from build123d import *

# Parameters (mm, degrees)
SKETCH1_R                = 14.312899999999999
BOSS_EXTRUDE1_DEPTH      = 6.35
FILLET1_R                = 14.2875
SKETCH2_W                = 63.5
SKETCH2_H                = 38.099999999999994
BOSS_EXTRUDE2_DEPTH      = 6.35
FILLET2_R                = 14.2875
SKETCH5_W                = 80.56082205671558
SKETCH5_H                = 59.96207335790194
CUT_EXTRUDE3_DEPTH       = 105.34114720473416
SKETCH6_R                = 14.312899999999999
BOSS_EXTRUDE3_DEPTH      = 88.89999999999999
CHAMFER1_SIZE            = 123.334861862
CHAMFER1_SIZE_2          = 86.36
CHAMFER2_START           = -41.62371919
CHAMFER2_OUTLINE_W       = 158.00000000000003
CHAMFER2_OUTLINE_H       = 88.9
CHAMFER2_DEPTH           = 70.741970545
BOSS_EXTRUDE4_DEPTH      = 6.35
BOSS_EXTRUDE5_DEPTH      = 73.65999999999998
CUT_EXTRUDE9_DEPTH       = 140.7047508401556
CUT_EXTRUDE9_DEPTH_BACK  = 140.7047508401556
CUT_EXTRUDE10_DEPTH      = 73.65999999999998
CUT_EXTRUDE10_DEPTH_BACK = 184.87947802715968
FILLET3_R                = 20.16
SKETCH19_R               = 2.539999999999996
CUT_EXTRUDE11_DEPTH      = 184.87947795602068
SKETCH20_R               = 2.5400000000000027
SKETCH20_R_2             = 2.540000000000001
CUT_EXTRUDE12_DEPTH      = 188.65942191717963
FILLET4_R                = 20.16
CUT_EXTRUDE13_DEPTH      = 330.8952367610784
CUT_EXTRUDE13_DEPTH_BACK = 330.8952367610784
SKETCH21_W               = 304.0212933781311
SKETCH21_H               = 127.80861110845143


with BuildPart() as part:
    # Sketch1 → Boss-Extrude1 (new body)
    with BuildSketch(Plane.XY):
        Polygon((-6.34999999999998, -6.349999999999993), (63.500000000000014, -6.349999999999988), (63.50000000000003, 44.44999999999999), (-63.49999999999997, 44.44999999999999), (-63.49999999999994, -44.45), (-31.749999999999943, -44.45), align=None)
        with Locations((-44.44999999999997, -25.400000000000006)):
            Circle(SKETCH1_R, mode=Mode.SUBTRACT)
        with Locations((35.87185256827684, 12.70000000000001)):
            Circle(SKETCH1_R, mode=Mode.SUBTRACT)
    extrude(amount=BOSS_EXTRUDE1_DEPTH)

    # Fillet1
    fillet1_edges = [part.edges().sort_by_distance(p)[0] for p in [
        (-31.749999999999943, -44.45, 3.175),
        (-63.49999999999994, -44.45, 3.175),
        (63.50000000000002, -6.349999999999987, 3.175),
        (-6.349999999999981, -6.349999999999993, 3.175),
    ]]
    fillet(fillet1_edges, radius=FILLET1_R)

    # Sketch2 → Boss-Extrude2 (add)
    with BuildSketch(Plane.XY.offset(6.35)):
        with Locations((2.842e-14, 63.499999999999986)):
            Rectangle(SKETCH2_W, SKETCH2_H)
    extrude(amount=-BOSS_EXTRUDE2_DEPTH)

    # Fillet2
    fillet2_edges = [part.edges().sort_by_distance(p)[0] for p in [
        (-31.74999999999997, 82.54999999999998, 3.175),
        (31.75000000000003, 82.54999999999998, 3.175),
        (31.75000000000003, 44.44999999999999, 3.175),
    ]]
    fillet(fillet2_edges, radius=FILLET2_R)

    # Sketch5 → Cut-Extrude3 (cut, through all)
    with BuildSketch(Plane.XY.offset(6.35)):
        with Locations((8.530411028357818, 74.43103667895096)):
            Rectangle(SKETCH5_W, SKETCH5_H)
    extrude(amount=-CUT_EXTRUDE3_DEPTH, mode=Mode.SUBTRACT)

    # Sketch6 → Boss-Extrude3 (add)
    # profile 1 of 2: a face of its own
    with BuildSketch(Plane.XY.offset(6.35)):
        with BuildLine():
            Line((-27.50851936904525, -38.08777905356794), (49.21250000000003, -6.349999999999989))
            Line((49.21250000000003, -6.349999999999989), (1.296437949397273, -6.3499999999999925))
            ThreePointArc((1.296437949397273, -6.3499999999999925), (-5.445232161641531, -8.040574170103001), (-10.591480630954672, -12.71222094643204))
            Line((-10.591480630954672, -12.71222094643204), (-27.50851936904525, -38.08777905356794))
        make_face()
    # profile 2 of 2: a face of its own
    with BuildSketch(Plane.XY.offset(6.35)):
        with BuildLine():
            ThreePointArc((49.21250000000003, -6.349999999999989), (59.315288136202824, -2.1652881362027863), (63.50000000000003, 7.937500000000011))
            Line((63.50000000000003, 7.937500000000011), (63.50000000000003, 44.44999999999999))
            Line((63.50000000000003, 44.44999999999999), (-63.49999999999997, 44.44999999999999))
            Line((-63.49999999999997, 44.44999999999999), (-63.49999999999994, -30.162500000000005))
            ThreePointArc((-63.49999999999994, -30.162500000000005), (-59.31528813620274, -40.2652881362028), (-49.21249999999995, -44.45))
            Line((-49.21249999999995, -44.45), (-39.396437949397196, -44.45))
            ThreePointArc((-39.396437949397196, -44.45), (-32.65476783835839, -42.759425829897), (-27.50851936904525, -38.08777905356794))
            Line((-27.50851936904525, -38.08777905356794), (-10.591480630954672, -12.71222094643204))
            ThreePointArc((-10.591480630954672, -12.71222094643204), (-5.445232161641531, -8.040574170103001), (1.296437949397273, -6.3499999999999925))
            Line((1.296437949397273, -6.3499999999999925), (49.21250000000003, -6.349999999999989))
        make_face()
        with Locations((35.87185256827684, 12.70000000000001)):
            Circle(SKETCH6_R, mode=Mode.SUBTRACT)
        with Locations((-44.44999999999997, -25.400000000000006)):
            Circle(SKETCH6_R, mode=Mode.SUBTRACT)
    extrude(amount=-BOSS_EXTRUDE3_DEPTH)

    # Chamfer1
    # the kernel refuses this chamfer: 123.334861862, 86.36 mm, written as the material it takes off along each edge
    with BuildSketch(Plane(origin=(63.50000000000003, -310.58122257411287, -82.55), x_dir=(-1, 0, 0), z_dir=(0, 1, 0))) as chamfer1_piece_1:
        Polygon((CHAMFER1_SIZE, 0), (0, CHAMFER1_SIZE_2), (0, 0), align=None)
    extrude(amount=673.5499451482258, mode=Mode.SUBTRACT)

    # Chamfer2: read off the stored shape, not the designer's step
    # Chamfer2 outline → Chamfer2 (cut)
    with BuildSketch(Plane(origin=(0, 0, 0), x_dir=(0.819152044288991, 0, 0.5735764363510472), z_dir=(0.5735764363510472, 0, -0.8191520442889911)).offset(CHAMFER2_START)):
        with Locations((-22.000000000000004, 0)):
            Rectangle(CHAMFER2_OUTLINE_W, CHAMFER2_OUTLINE_H)
    extrude(amount=CHAMFER2_DEPTH, mode=Mode.SUBTRACT)

    # Sketch8 → Boss-Extrude4 (add)
    with BuildSketch(Plane(origin=(63.50000000000003, 0, 0), x_dir=(0, 0, -1), z_dir=(1, 0, 0))):
        Polygon((-3.8100000000002296, 44.44999999999999), (-41.91000000000023, 44.44999999999998), (-41.910000000000224, 7.937500000000005), (-3.8100000000002257, 7.937500000000011), align=None)
    extrude(amount=-BOSS_EXTRUDE4_DEPTH)

    # Sketch10 → Boss-Extrude5 (add)
    with BuildSketch(Plane(origin=(0, 44.44999999999999, 0), x_dir=(1, 0, 0), z_dir=(0, 1, 0))):
        Polygon((-57.84497848897024, 130.81000000000014), (-63.49999999999997, 130.81000000000014), (-63.49999999999997, 80.01000000000018), (-57.844978488970234, 80.01000000000016), align=None)
    extrude(amount=-BOSS_EXTRUDE5_DEPTH)

    # Sketch17 → Cut-Extrude9 (cut, two sides: drawn at the far end of the back side and taken through both)
    with BuildSketch(Plane(origin=(19.10074600681286, 0, -27.278692336917096), x_dir=(-0.8191520442889909, 0, -0.5735764363510474), z_dir=(0.5735764363510474, 0, -0.8191520442889909)).offset(-CUT_EXTRUDE9_DEPTH_BACK)):
        with BuildLine():
            add(Edge.make_bspline(
                [(94.42353448054058, -29.21), (95.93788750756819, -24.718047698019056), (93.93338517829203, -20.356820676396385)],
                knots=[2.872150837356143, 2.872150837356143, 2.872150837356143, 3.5016757767347815, 3.5016757767347815, 3.5016757767347815], degree=2, weights=[1, 0.9508699428937519, 1]))
            add(Edge.make_bspline(
                [(93.93338517829203, -20.356820676396385), (88.79622683458668, -9.179825042266891), (74.45226902252679, -11.318450120374129), (60.108311210466894, -13.457075198481366), (60.108311210466894, -25.4)],
                knots=[3.5016757767347815, 3.5016757767347815, 3.5016757767347815, 4.892430541957184, 4.892430541957184, 6.283185307179586, 6.283185307179586, 6.283185307179586], degree=2, weights=[1, 0.7678119767762641, 1, 0.7678119767762641, 1]))
            add(Edge.make_bspline(
                [(60.108311210466894, -25.400000000000002), (60.108311210466894, -37.903779229296156), (75.2342951684929, -39.58320874739981), (90.36027912651893, -41.262638265503455), (94.42353448054058, -29.21)],
                knots=[0, 0, 0, 1.4360754186780715, 1.4360754186780715, 2.872150837356143, 2.872150837356143, 2.872150837356143], degree=2, weights=[1, 0.7530981852489751, 1, 0.7530981852489751, 1]))
        make_face()
    extrude(amount=CUT_EXTRUDE9_DEPTH + CUT_EXTRUDE9_DEPTH_BACK, mode=Mode.SUBTRACT)

    # Sketch18 → Cut-Extrude10 (cut, two sides: drawn at the far end of the back side and taken through both)
    with BuildSketch(Plane(origin=(-57.84497848897023, 0, 7.9e-15), x_dir=(-1.4e-16, 0, -1), z_dir=(1, 0, -1.4e-16)).offset(-CUT_EXTRUDE10_DEPTH_BACK)):
        Polygon((130.81000000000014, -29.21), (81.15666866187213, -29.210000000000008), (81.15666866187213, -3.8100000000000076), (130.81000000000014, -3.810000000000001), align=None)
    extrude(amount=CUT_EXTRUDE10_DEPTH + CUT_EXTRUDE10_DEPTH_BACK, mode=Mode.SUBTRACT)

    # Fillet3
    # the kernel refuses this fillet: 20.16 mm, written as the material it adds along each edge
    with BuildSketch(Plane(origin=(57.150000000000034, 44.44999999999999, 4.470039485332174), x_dir=(-0.8191520442889912, 0, -0.5735764363510469), z_dir=(0, -1, 0))) as fillet3_piece_1_section:
        with BuildLine():
            CenterArc((FILLET3_R * 0.520567050552, -FILLET3_R), FILLET3_R, 90.00000000000001, 54.99999999999993)
            Line((-FILLET3_R * 0.298584993737, -FILLET3_R * 0.426423563649), (0, 0))
            Line((0, 0), (FILLET3_R * 0.520567050552, 0))
        make_face()
    fillet3_piece_1 = extrude(amount=36.51249999999998, mode=Mode.PRIVATE)
    fillet3_piece_1 = fillet3_piece_1 - Plane(origin=(35.87185256827684, 12.70000000000001, 4.470039485332174), x_dir=(1, 0, 0), z_dir=(0, 0, 1)) * Cylinder(14.312899999999999, 116, mode=Mode.PRIVATE)
    add(fillet3_piece_1)
    with BuildSketch(Plane(origin=(-57.844978488970234, 44.44999999999999, -81.15666866204359), x_dir=(0.8191520442884476, 0, 0.5735764363518233), z_dir=(0, -1, 0))) as fillet3_piece_2:
        with BuildLine():
            CenterArc((FILLET3_R * 0.520567050551, -FILLET3_R), FILLET3_R, 90.00000000000001, 54.99999999994567)
            Line((-FILLET3_R * 0.298584993737, -FILLET3_R * 0.426423563648), (0, 0))
            Line((0, 0), (FILLET3_R * 0.520567050551, 0))
        make_face()
    extrude(amount=48.25999999999999)

    # Sketch19 → Cut-Extrude11 (cut, through all)
    with BuildSketch(Plane(origin=(-57.84497848897023, 0, 7.9e-15), x_dir=(-1.4e-16, 0, -1), z_dir=(1, 0, -1.4e-16))):
        with Locations((121.28500000000014, 28.57499999999999)):
            Circle(SKETCH19_R)
        with Locations((121.28500000000014, 5.7149999999999945)):
            Circle(SKETCH19_R)
    extrude(amount=-CUT_EXTRUDE11_DEPTH, mode=Mode.SUBTRACT)

    # Sketch20 → Cut-Extrude12 (cut, through all)
    with BuildSketch(Plane(origin=(63.50000000000003, 0, 0), x_dir=(0, 0, -1), z_dir=(1, 0, 0))):
        with Locations((-32.38500000000023, 25.39999999999998)):
            Circle(SKETCH20_R)
        with Locations((-16.510000000000232, 25.399999999999977)):
            Circle(SKETCH20_R_2)
    extrude(amount=-CUT_EXTRUDE12_DEPTH, mode=Mode.SUBTRACT)

    # Fillet4
    # the kernel refuses this fillet: 20.16 mm, written as the material it takes off along each edge
    with BuildSketch(Plane(origin=(-41.42329156376277, -29.209999999999994, -82.55), x_dir=(0, -2.04e-14, 1), z_dir=(-1, 0, 0))) as fillet4_piece_1:
        with BuildLine():
            CenterArc((20.160000000000146, -7.364628119294481), FILLET4_R, 158.57340370727903, 21.426596292722138)
            Line((1.5023e-13, -7.364628119294892), (-0.403199999999848, -7.3646281192949))
            Line((-0.403199999999848, -7.3646281192949), (-0.4031999999999982, -8.22e-15))
            Line((-0.4031999999999982, -8.22e-15), (-8.22e-15, 0.4031999999999982))
            ThreePointArc((-8.22e-15, 0.4031999999999982), (0.6966656690639528, 0.4031999999999982), (1.0179979648904802, 0.14729256238588861))
            Line((1.0179979648904802, 0.14729256238588861), (1.393331338127922, 0))
        make_face()
    extrude(amount=40.48827873447443, mode=Mode.SUBTRACT)

    # Mirror1: part across plane


with BuildPart() as part_1:
    add(part.part)
    add(part.part.mirror(Plane(origin=(-57.84497848897024, -29.21, -130.81000000000014), x_dir=(1, 0, 0), z_dir=(0, 0, -1))))

    # Sketch21 → Cut-Extrude13 (cut, two sides: drawn at the far end of the back side and taken through both)
    with BuildSketch(Plane(origin=(-57.84497848897023, 0, 7.9e-15), x_dir=(-1.4e-16, 0, -1), z_dir=(1, 0, -1.4e-16)).offset(-CUT_EXTRUDE13_DEPTH_BACK)):
        with Locations((-21.20064668906538, -19.454305554225726)):
            Rectangle(SKETCH21_W, SKETCH21_H)
    extrude(amount=CUT_EXTRUDE13_DEPTH + CUT_EXTRUDE13_DEPTH_BACK, mode=Mode.SUBTRACT)


solid = part_1.part
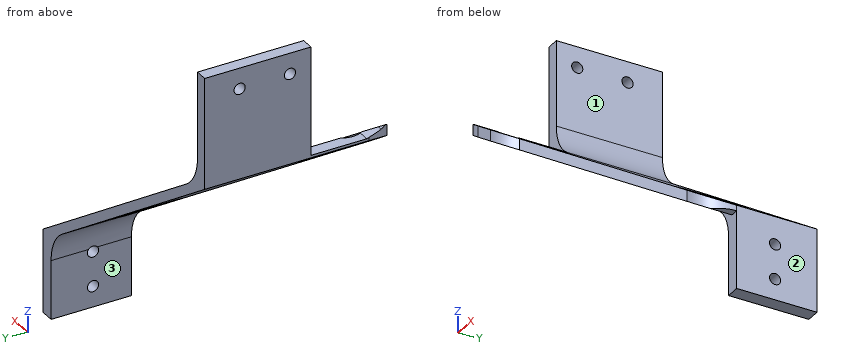
Geometry: final body of the model. Coordinates: model frame, mm. Face numbers are marked on the shaded views. A direction names the side the tool comes from. Give positions to 0.01 mm unless a question says otherwise; leave off trailing zeros. Loops run counter-clockwise (first coordinate to the right, second up) from the corner with the lowest first, then second, coordinate; pieces in that order, holes last. Notation, with made-up numbers: (-39.5, 36.5) - (-33.5, 36.5) arc R32 cw to (-33.5, 74.5) - close; hole circle Ø5 at (62.5, 85). An arc over 180 degrees is marked (long way). Answer as CSV lines item,"result". Start each with the question number.
1. Pin query (flat end, axial travel): P1, Ø2, axis at x = -18, y = 26, coming from the -Z side; P2, Ø3, axis at x = 62.5, y = 4.5, coming from the -Z side; P3, Ø3, axis at x = -60.5, y = -22, coming from the +Z side; P4, Ø17, axis at x = 35.87, y = 12.7, coming from the -Z side. Return the tip coordinate at first contact, or that it passes through.
2. Section B-B, the plane x = 38. Return loops of the section in (y, z), plus the area to 3 significant figures.
3. Section C-C, the plane z = -250.5. Return loops of the section in (x, y), plus the area to 3 significant figures.
4. Ray query, L1, parallel to Y at x = 62.25, z = -278.13; L2, parallel to Y at x = -44, z = -193; L3, parallel to Z at x = 60.5, y = 25.4 (3 decimals). Return the intervals inside material, ascending.
5. Reachability of the marked faces 1, 2 and 3 from +Z, -Z, +X, -X, +Y, -Y: full face, straight path, thin tool, end or side. Return the list, or none.
6. Section D-D, the plane y = 12.7. Return loops of the section in (x, z), plus the area to 3 significant figures.
7. Section A-A, the plane y = 37. Return loops of the section in (x, z).
Answers:
1,P1,"stops at z = -214.17"
1,P2,"stops at z = -267.97"
1,P3,"stops at z = -180.46"
1,P4,"passes through"
2,outline,"(-10.99, -252.68) - (-1.45, -252.68) - (-1.45, -247.57) - (-10.99, -247.57) - close; (26.85, -252.68) - (44.45, -252.68) - (44.45, -247.57) - (26.85, -247.57) - close"
2,area,"139 mm2"
3,outline,"(34.89, -12.28) - (42.18, -9.26) - (42.18, -0.15) arc R14.31 cw to (34.89, -1.58) - close; (34.89, 26.98) arc R14.31 cw to (42.18, 25.55) - (42.18, 44.45) - (34.89, 44.45) - close"
3,area,"200 mm2"
4,L1,"y = 7.94 to 22.86, 27.94 to 44.45"
4,L2,"y = -44.45 to -39.71, -11.09 to 44.45"
4,L3,"z = -303.53 to -296.545, -291.465 to -280.67, -275.59 to -263.329"
5,face 1,"+Z, +X, +Y, -Y"
5,face 2,"+Z, -Z, +X, +Y, -Y"
5,face 3,"-Z, -X, +Y, -Y"
6,outline,"(-63.5, -181.61) - (21.56, -241.17) - (21.56, -236.06) - (-49.25, -186.48) arc R20.16 cw to (-57.84, -169.97) - (-57.84, -130.81) - (-63.5, -130.81) - close; (50.18, -261.34) arc R20.16 cw to (57.15, -276.58) - (57.15, -303.53) - (63.5, -303.53) - (63.5, -265.43) - (50.18, -256.11) - close"
6,area,"1,030 mm2"
7,outline,"(-63.5, -181.61) - (48.55, -260.07) arc R20.16 cw to (57.15, -276.58) - (57.15, -303.53) - (63.5, -303.53) - (63.5, -265.43) - (-49.25, -186.48) arc R20.16 cw to (-57.84, -169.97) - (-57.84, -130.81) - (-63.5, -130.81) - close"
